The listing builds one solid part. Answer for the finished solid, in the listing's coordinates (mm). Face numbers are marked on the shaded views. A direction names the side the tool comes from. Round coordinates to 2 decimals unless told otherwise and drop trailing zeros. Write each loop counter-clockwise with the first axis right and the second up, starting at its lowest first coordinate (ties: lowest second). Pieces come first, ordered by that corner, then holes. Notation, with made-up numbers: M 48,76 L 68,76 A24 cw 68,114 Z; hole C 48.25,4 d9. An arc over 180 degrees is marked long. One line per item, written item: value. Start each with the question number.
(1) Given P1, Ø1.5, axis at y = -11.5, z = -2.5, coming from the -X side; P2, Ø3, axis at y = -2, z = -0.5, coming from the -X side; P3, Ø1.5, axis at x = -58, z = -3.5, coming from the -Y side, each flat-ended and moving along its own axis, determine where each tip first touches the part or whether it passes through.
(2) Consider probe 1 along X at (y, z) = (2.9, -3); probe 2 along X at (y, z) = (2.5, -2.5); probe 3 along Y at (x, z) = (-78, -0.15). Determine where each line is inside the solid, lowest interval first.
(3) Section A-A (z = -3) is taken. Determine the outline of the cut face in (x, y), plus the area to 3 significant figures.
(4) Section C-C (x = -46.5) is taken. Determine the outline of the cut face in (y, z).
(5) Section B-B (y = -12.5) is taken. Determine the outline of the cut face in (x, z), plus the area to 3 significant figures.
(6) For the marked faces 1 and 2, determine the directions among +Z, -Z, +X, -X, +Y, -Y from which every point of the face is accessible in a straight line to the end or side of a thin tool.
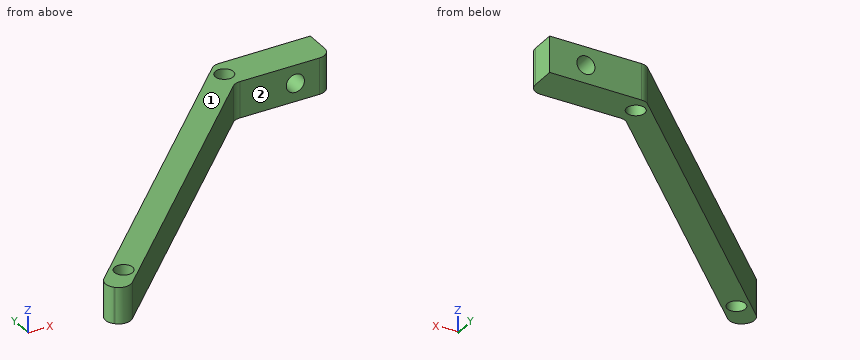
```python
from build123d import *

# Parameters (mm, degrees)
F1_DEPTH = 6
F0_R     = 1.5
F2_DEPTH = 6
F3_R     = 1.5
F4_DEPTH = 12.5
F5_R     = 2


with BuildPart() as f1:
    # F0 (on Top) → F1 (new body)
    with BuildSketch(Plane.XY):
        with BuildLine():
            Line((-20.562754872, -1.2907197386), (-20.562754872, 4.7092802614))
            Line((-20.562754872, 4.7092802614), (-36.5625023842, 4.6193939634))
            Line((-36.5625023842, 4.6193939634), (-36.5625023842, 3.1643371124))
            ThreePointArc((-36.5625023842, 3.1643371124), (-35.0625023842, 1.6643371124), (-36.5625023842, 0.1643371124))
            Line((-36.5625023842, 0.1643371124), (-36.5625023842, -1.2907197386))
            Line((-36.5625023842, -1.2907197386), (-20.562754872, -1.2907197386))
        make_face()
    extrude(amount=-F1_DEPTH)

    # F0 (on Top) → F2 (join)
    with BuildSketch(Plane.XY):
        with BuildLine():
            Line((-36.5625023842, 3.1643371124), (-36.5625023842, 4.6193939634))
            Line((-36.5625023842, 4.6193939634), (-81.9439661063, -40.7620697588))
            Line((-81.9439661063, -40.7620697588), (-78.9889092554, -43.7171266098))
            Line((-78.9889092554, -43.7171266098), (-36.5625023842, -1.2907197386))
            Line((-36.5625023842, -1.2907197386), (-36.5625023842, 0.1643371124))
            ThreePointArc((-36.5625023842, 0.1643371124), (-38.0625023842, 1.6643371124), (-36.5625023842, 3.1643371124))
        make_face()
        with Locations((-76.8675889118, -38.6407494152)):
            Circle(F0_R, mode=Mode.SUBTRACT)
    extrude(amount=-F2_DEPTH)

    # F3 (on Front) → F4 (cut, symmetric)
    with BuildSketch(Plane.XZ):
        with Locations((-26.562754872, -3)):
            Circle(F3_R)
    extrude(amount=F4_DEPTH, both=True, mode=Mode.SUBTRACT)

    # F5
    f5_edges = [f1.edges().sort_by_distance(p)[0] for p in [
        (-36.562502, 4.619394, -3),
        (-20.562755, -1.29072, -3),
        (-36.562502, -1.29072, -3),
        (-78.988909, -43.717127, -3),
        (-81.943966, -40.76207, -3),
    ]]
    fillet(f5_edges, radius=F5_R)


solid = f1.part
```
Recorded:
1. P1: stops at x = -53.43
1. P2: stops at x = -44.68
1. P3: stops at y = -23.48
2. probe 1: x = -38.28 to -37.41, -35.71 to -28.06, -25.06 to -20.56
2. probe 2: x = -38.68 to -37.81, -35.32 to -27.98, -25.15 to -20.56
2. probe 3: y = -42.63 to -39.62, -37.66 to -36.82
3. outline: M -80.53,-42.18 L -80.4,-42.3 A2 ccw -77.57,-42.3 L -37.15,-1.88 A2 cw -35.73,-1.29 L -28.06,-1.29 L -28.06,4.67 L -35.74,4.62 A2 ccw -37.14,4.04 L -80.53,-39.35 A2 ccw Z; M -25.06,-1.29 L -22.56,-1.29 A2 ccw -20.56,0.71 L -20.56,4.71 L -25.06,4.68 Z; hole C -76.87,-38.64 d3; hole C -36.56,1.66 d3
3. area: 320 mm2
4. outline: M -11.23,-6 L -5.32,-6 L -5.32,0 L -11.23,0 Z
5. outline: M -53.68,-6 L -47.77,-6 L -47.77,0 L -53.68,0 Z
5. area: 35.5 mm2
6. face 1: +Z, +X, -X, +Y, -Y
6. face 2: +Z, -Z, +X, -Y
